Part model, mm, in its own coordinate system. A direction names the side the tool comes from. Round coordinates to 2 decimals unless told otherwise and drop trailing zeros. Write each loop counter-clockwise with the first axis right and the second up, starting at its lowest first coordinate (ties: lowest second). Pieces come first, ordered by that corner, then holes. Notation, with made-up numbers: M 45.5,68 L 87.5,68 A37 ccw 87.5,106 Z; hole C 70,39 d1. An arc over 180 degrees is marked long. Answer as a JSON object with one key per item and string values. Group by question number.
1. Which spindle directions (+Z, -Z, +X, -X, +Y, -Y) get a long thin tool onto all of the face, cutting with end or side? Do faces 1 (the face through (0, 0, 0)), 2 (the face through (-0.931, -28.933, -2.957)). Say none if no direction does.
2. Band-saw the part on A-A, the plane y = -42. Write the cut outline in (x, z).
3. Drop flat-ended pins along their axis: pin 1 (4 mm diameter, centred on x = 3, y = -35, fed in from -Z); pin 2 (2 mm diameter, centred on y = -29.5, z = -3, fed in from +X); pin 3 (1.5 mm diameter, centred on x = -2.5, y = -20.5, fed in from -Z). Give the stop position or say it passes through.
4. Drill centre lines: line 1 (X direction, y = -14.5, z = 0.25); line 2 (Y direction, x = 0, z = 1.75). Where is each one in solid material? Low to high. Write a range as from..to.
from build123d import *

# Parameters (mm, degrees)
CUT_EXTRUDE1_DEPTH = 56.489098028
CIRPATTERN1_COUNT  = 3


with BuildPart() as part:
    # Sketch1 → Revolve1 (revolve)
    with BuildSketch(Plane.XY, mode=Mode.PRIVATE) as revolve1_sk:
        Polygon((0, 0), (4, 0), (4, -0.5), (3.1, -2.058845727), (3.1, -55.2), (0, -55.2), align=None)
    revolve(revolve1_sk.sketch.rotate(Axis((0, -60.2, 0), (0, 1, 0)), 90), axis=Axis((0, -60.2, 0), (0, 1, 0)))

    # Sketch2 → Cut-Extrude1 (cut, symmetric)
    with BuildSketch(Plane.XY):
        Polygon((0, -55.2), (3.1, -55.2), (3.1, -54.928785143), align=None)
    cut_extrude1 = extrude(amount=CUT_EXTRUDE1_DEPTH, both=True, mode=Mode.SUBTRACT)

    # CirPattern1: Cut-Extrude1 ×3 about axis
    cirpattern1_axis = Axis((0, 0, 0), (0, 1, 0))
    for i in range(1, CIRPATTERN1_COUNT):
        add(cut_extrude1.rotate(cirpattern1_axis, i * 360 / CIRPATTERN1_COUNT), mode=Mode.SUBTRACT)


solid = part.part
Worked answers:
{
 "1": {"face 1": "+Z, -Z, +X, -X, +Y", "face 2": "-Y"},
 "2": {"outline": "C 0,0 d6.2"},
 "3": {"pin 1": "stops at z = -2.93", "pin 2": "stops at x = 2.37", "pin 3": "stops at z = -2.56"},
 "4": {"line 1": "x = -3.09..3.09", "line 2": "y = -55.07..0"}
}
